```python
from build123d import *

# Parameters (mm, degrees)
BOSS_EXTRUDE6_DEPTH = 18.288
BOSS_EXTRUDE7_DEPTH = 2.54
SKETCH4_R           = 1.905
CUT_EXTRUDE2_DEPTH  = 51.8
FILLET2_R           = 2.54


with BuildPart() as part:
    # Sketch3 → Boss-Extrude6 (new body)
    with BuildSketch(Plane.XY):
        with BuildLine():
            Line((25.4, 30.988), (25.4, 0))
            Line((25.4, 0), (29.718, 0))
            Line((29.718, 0), (29.718, 29.480573053))
            ThreePointArc((29.718, 29.480573053), (43.434, 46.99), (29.718, 64.499426947))
            Line((29.718, 64.499426947), (29.718, 82.55))
            Line((29.718, 82.55), (25.4, 82.55))
            Line((25.4, 82.55), (25.4, 62.992))
            ThreePointArc((25.4, 62.992), (36.715122713, 58.305122713), (41.402, 46.99))
            ThreePointArc((41.402, 46.99), (36.715122713, 35.674877287), (25.4, 30.988))
        make_face()
    extrude(amount=BOSS_EXTRUDE6_DEPTH)

    # Sketch3_10 → Boss-Extrude7 (add)
    with BuildSketch(Plane.XY):
        with BuildLine():
            Line((29.718, 29.480573053), (29.718, 0))
            Line((29.718, 0), (50.8, 0))
            Line((50.8, 0), (50.8, 82.55))
            Line((50.8, 82.55), (29.718, 82.55))
            Line((29.718, 82.55), (29.718, 64.499426947))
            ThreePointArc((29.718, 64.499426947), (43.434, 46.99), (29.718, 29.480573053))
        make_face()
    extrude(amount=BOSS_EXTRUDE7_DEPTH)

    # Sketch4 → Cut-Extrude2 (cut, through all)
    with BuildSketch(Plane(origin=(0, 0, 0), x_dir=(0, 0, -1), z_dir=(1, 0, 0))):
        with Locations((-11.684, 14.740286527)):
            Circle(SKETCH4_R)
        with Locations((-11.684, 73.524713473)):
            Circle(SKETCH4_R)
    extrude(amount=CUT_EXTRUDE2_DEPTH, mode=Mode.SUBTRACT)

    # Fillet2
    fillet2_edges = [part.edges().sort_by_distance(p)[0] for p in [
        (43.434, 46.99, 2.54),
        (29.718, 14.740286527, 2.54),
        (29.718, 73.524713473, 2.54),
    ]]
    fillet(fillet2_edges, radius=FILLET2_R)


solid = part.part
```
Here's how the part is built. I have some questions about the finished solid (model axes, mm). A direction names the side the tool comes from. Give positions to 0.01 mm unless a question says otherwise; leave off trailing zeros. Write each loop counter-clockwise with the first axis right and the second up, starting at its lowest first coordinate (ties: lowest second). Pieces come first, ordered by that corner, then holes.
(1) Imagine slicing it at A-A, the plane z = 1.5. Write out the boundary of the cut face in (x, y).
Output values:
outline: (25.4, 0) - (50.8, 0) - (50.8, 82.55) - (25.4, 82.55) - (25.4, 62.99) arc R16 cw to (25.4, 30.99) - close
(2) Imagine slicing it at D-D, the plane z = 15.5. Write out the boundary of the cut face in (x, y).
Output values:
outline: (25.4, 0) - (29.72, 0) - (29.72, 29.48) arc R18.03 ccw to (29.72, 64.5) - (29.72, 82.55) - (25.4, 82.55) - (25.4, 62.99) arc R16 cw to (25.4, 30.99) - close
(3) Imagine slicing it at C-C, the plane y = 20. Write out the boundary of the cut face in (x, z), and give its area (3 significant figures).
Output values:
outline: (25.4, 0) - (50.8, 0) - (50.8, 2.54) - (32.26, 2.54) arc R2.54 cw to (29.72, 5.08) - (29.72, 18.29) - (25.4, 18.29) - close
area: 134 mm2
(4) Imagine slicing it at B-B, the plane z = 11.5. Write out the boundary of the cut face in (x, y).
Output values:
outline: (25.4, 0) - (29.72, 0) - (29.72, 12.84) - (25.4, 12.84) - close; (25.4, 16.64) - (29.72, 16.64) - (29.72, 29.48) arc R18.03 ccw to (29.72, 64.5) - (29.72, 71.63) - (25.4, 71.63) - (25.4, 62.99) arc R16 cw to (25.4, 30.99) - close; (25.4, 75.42) - (29.72, 75.42) - (29.72, 82.55) - (25.4, 82.55) - close
(5) Will these pins go through, and if not, where does the flat tip stop? pin 1 (2.5 mm diameter, centred on y = 14.74, z = 11.68, fed in from +X); pin 2 (1 mm diameter, centred on y = 43, z = 9, fed in from +X); pin 3 (10.5 mm diameter, centred on y = 14, z = 14, fed in from +X); pin 4 (5 mm diameter, centred on x = 36.5, z = 13.5, fed in from +Y).
Output values:
pin 1: passes through
pin 2: stops at x = 43.09
pin 3: stops at x = 29.72
pin 4: stops at y = 62.84
(6) If I drill on L1, parallel to Z at x = 47, y = 22.5; L2, parallel to Y at x = 30.5, z = 2; L3, parallel to Y at x = 27, z = 17, over which ranges is the centre line in solid material (lowest first)?
Output values:
L1: z = 0 to 2.54
L2: y = 0 to 31.82, 62.16 to 82.55
L3: y = 0 to 31.07, 62.91 to 82.55
(7) On a 3-axis mill with a long thin cutter (end or side, diameter ignored), from which of +Z, -Z, +X, -X, +Y, -Y can I reach the whole of each face in a straight line? I mean faces 5 (the face through (43.43, 46.65, 11.59)), 6 (the face through (30.482, 73.398, 3.264)), 7 (the face through (29.718, 15, 15)), 8 (the face through (25.4, 73, 9)). Say none if no direction works.
Output values:
face 5: +Z, +X
face 6: +Z, +X, +Y
face 7: +Z, +X, -Y
face 8: +Z, -Z, -X, +Y, -Y
(8) Thinking about a two-plate mould opening in Z: for faces 1 (the face through (41, 42, 0)), 2 (the face through (27.529, 13.05, 10.805)), 3 (the face through (30.5, 0, 3)), 4 (the face through (37, 35, 18.288)), which applies, pulls with the +Z half, pulls with the -Z half, needs draft (parallel to the pull), parting line crosses it, or undercut?
Output values:
face 1: pulls with the -Z half
face 2: undercut
face 3: needs draft
face 4: pulls with the +Z half
